Read the model definition and answer for the solid it produces. Units are mm, in the model's axes. Coordinates: 2 decimals unless noted, no trailing zeros. Write each loop counter-clockwise with the first axis right and the second up, starting at its lowest first coordinate (ties: lowest second). Pieces come first, ordered by that corner, then holes. Notation, with made-up numbers: (75.25, 21.5) -> (107.25, 21.5) arc R21 ccw to (107.25, 59.5) -> close; hole circle Ø8 at (31.5, 80). An arc over 180 degrees is marked (long way). Answer in a Markdown table with one row per item. Add a question column.
Item 1: Straight lines are drawn through the part: line 1 (Y direction, x = 54, z = 1.4); line 2 (Y direction, x = 134, z = 1.4); line 3 (Y direction, x = 182, z = 1.25). For each, find the intervals that lie inside material, in ascending order. Write a range as from..to.
Item 2: Section B-B on y = 72 is taken. Count the separate pieces of the cut face and the enclosed holes in it, then the cut area to 3 significant figures.
Item 3: Given pin 1 Ø1.5 at (x, z) = (89, 1) entering from -Y; pin 2 Ø1.5 at (y, z) = (1, 1.5) entering from +X; pin 3 Ø0.9 at (y, z) = (15.5, 1) entering from -X, each flat-ended and moving along its own axis, determine where each tip first touches the part or whether it passes through.
Item 4: For a pull along Y with two mould halves and no side action, classify faces 1 (the face through (108, 152, 3)), 2 (the face through (21.479, 35.966, 1.521)) as +Y half, -Y half, draft (parallel to the pull), parting line (faces both ways), or undercut.
Item 5: Section A-A on x = 77 is taken. Write down the section's boundary in (y, z).
Item 6: Section D-D on x = 165 is taken. Write down the section's boundary in (y, z), then the cut area to 3 significant figures.
```python
from build123d import *

# Parameters (mm, degrees)
SKETCH_W      = 220
SKETCH_H      = 300
PAD_DEPTH     = 3
SKETCH001_R   = 7.5
SKETCH001_R_2 = 4
SKETCH001_W   = 20
SKETCH001_H   = 3
SKETCH001_W_2 = 3
SKETCH001_H_2 = 20
SKETCH001_H_3 = 17
POCKET_DEPTH  = 5


with BuildPart() as part:
    # Sketch → Pad (new body)
    with BuildSketch(Plane.XY):
        with Locations((110, 150)):
            Rectangle(SKETCH_W, SKETCH_H)
    extrude(amount=PAD_DEPTH)

    # Sketch001 (on Face6 of Pad) → Pocket (cut)
    with BuildSketch(Plane.XY.offset(3)):
        with Locations((33, 72)):
            Circle(SKETCH001_R)
        with Locations((55, 72)):
            Circle(SKETCH001_R)
        with Locations((77, 72)):
            Circle(SKETCH001_R)
        with Locations((99, 72)):
            Circle(SKETCH001_R)
        with Locations((121, 72)):
            Circle(SKETCH001_R)
        with Locations((143, 72)):
            Circle(SKETCH001_R)
        with Locations((165, 72)):
            Circle(SKETCH001_R)
        with Locations((187, 72)):
            Circle(SKETCH001_R)
        with Locations((22, 48)):
            Circle(SKETCH001_R_2)
        with Locations((38, 48)):
            Circle(SKETCH001_R_2)
        with Locations((54, 48)):
            Circle(SKETCH001_R_2)
        with Locations((70, 48)):
            Circle(SKETCH001_R_2)
        with Locations((86, 48)):
            Circle(SKETCH001_R_2)
        with Locations((102, 48)):
            Circle(SKETCH001_R_2)
        with Locations((118, 48)):
            Circle(SKETCH001_R_2)
        with Locations((134, 48)):
            Circle(SKETCH001_R_2)
        with Locations((150, 48)):
            Circle(SKETCH001_R_2)
        with Locations((166, 48)):
            Circle(SKETCH001_R_2)
        with Locations((182, 48)):
            Circle(SKETCH001_R_2)
        with Locations((198, 48)):
            Circle(SKETCH001_R_2)
        with Locations((22, 32)):
            Circle(SKETCH001_R_2)
        with Locations((38, 32)):
            Circle(SKETCH001_R_2)
        with Locations((54, 32)):
            Circle(SKETCH001_R_2)
        with Locations((70, 32)):
            Circle(SKETCH001_R_2)
        with Locations((86, 32)):
            Circle(SKETCH001_R_2)
        with Locations((102, 32)):
            Circle(SKETCH001_R_2)
        with Locations((118, 32)):
            Circle(SKETCH001_R_2)
        with Locations((134, 32)):
            Circle(SKETCH001_R_2)
        with Locations((150, 32)):
            Circle(SKETCH001_R_2)
        with Locations((166, 32)):
            Circle(SKETCH001_R_2)
        with Locations((182, 32)):
            Circle(SKETCH001_R_2)
        with Locations((198, 32)):
            Circle(SKETCH001_R_2)
        with Locations((22, 16)):
            Circle(SKETCH001_R_2)
        with Locations((38, 16)):
            Circle(SKETCH001_R_2)
        with Locations((54, 16)):
            Circle(SKETCH001_R_2)
        with Locations((70, 16)):
            Circle(SKETCH001_R_2)
        with Locations((86, 16)):
            Circle(SKETCH001_R_2)
        with Locations((102, 16)):
            Circle(SKETCH001_R_2)
        with Locations((118, 16)):
            Circle(SKETCH001_R_2)
        with Locations((134, 16)):
            Circle(SKETCH001_R_2)
        with Locations((150, 16)):
            Circle(SKETCH001_R_2)
        with Locations((166, 16)):
            Circle(SKETCH001_R_2)
        with Locations((182, 16)):
            Circle(SKETCH001_R_2)
        with Locations((198, 16)):
            Circle(SKETCH001_R_2)
        with Locations((10, 1.5)):
            Rectangle(SKETCH001_W, SKETCH001_H)
        with Locations((50, 1.5)):
            Rectangle(SKETCH001_W, SKETCH001_H)
        with Locations((90, 1.5)):
            Rectangle(SKETCH001_W, SKETCH001_H)
        with Locations((130, 1.5)):
            Rectangle(SKETCH001_W, SKETCH001_H)
        with Locations((170, 1.5)):
            Rectangle(SKETCH001_W, SKETCH001_H)
        with Locations((210, 1.5)):
            Rectangle(SKETCH001_W, SKETCH001_H)
        with Locations((10, 298.5)):
            Rectangle(SKETCH001_W, SKETCH001_H)
        with Locations((50, 298.5)):
            Rectangle(SKETCH001_W, SKETCH001_H)
        with Locations((90, 298.5)):
            Rectangle(SKETCH001_W, SKETCH001_H)
        with Locations((130, 298.5)):
            Rectangle(SKETCH001_W, SKETCH001_H)
        with Locations((170, 298.5)):
            Rectangle(SKETCH001_W, SKETCH001_H)
        with Locations((210, 298.5)):
            Rectangle(SKETCH001_W, SKETCH001_H)
        with Locations((1.5, 50)):
            Rectangle(SKETCH001_W_2, SKETCH001_H_2)
        with Locations((1.5, 90)):
            Rectangle(SKETCH001_W_2, SKETCH001_H_2)
        with Locations((1.5, 130)):
            Rectangle(SKETCH001_W_2, SKETCH001_H_2)
        with Locations((1.5, 170)):
            Rectangle(SKETCH001_W_2, SKETCH001_H_2)
        with Locations((1.5, 210)):
            Rectangle(SKETCH001_W_2, SKETCH001_H_2)
        with Locations((1.5, 250)):
            Rectangle(SKETCH001_W_2, SKETCH001_H_2)
        with Locations((218.5, 50)):
            Rectangle(SKETCH001_W_2, SKETCH001_H_2)
        with Locations((218.5, 90)):
            Rectangle(SKETCH001_W_2, SKETCH001_H_2)
        with Locations((218.5, 130)):
            Rectangle(SKETCH001_W_2, SKETCH001_H_2)
        with Locations((218.5, 170)):
            Rectangle(SKETCH001_W_2, SKETCH001_H_2)
        with Locations((218.5, 210)):
            Rectangle(SKETCH001_W_2, SKETCH001_H_2)
        with Locations((218.5, 250)):
            Rectangle(SKETCH001_W_2, SKETCH001_H_2)
        with Locations((1.5, 11.51)):
            Rectangle(SKETCH001_W_2, SKETCH001_H_3)
        with Locations((1.5, 288.5)):
            Rectangle(SKETCH001_W_2, SKETCH001_H_3)
        with Locations((218.5, 288.5)):
            Rectangle(SKETCH001_W_2, SKETCH001_H_3)
        with Locations((218.5, 11.51)):
            Rectangle(SKETCH001_W_2, SKETCH001_H_3)
    extrude(amount=-POCKET_DEPTH, mode=Mode.SUBTRACT)


solid = part.part
```
Results below:
| question | item | result |
|---|---|---|
| 1 | line 1 | y = 3..12, 20..28, 36..44, 52..64.57, 79.43..297 |
| 1 | line 2 | y = 3..12, 20..28, 36..44, 52..297 |
| 1 | line 3 | y = 0..12, 20..28, 36..44, 52..66.41, 77.59..300 |
| 2 | separate pieces | 9 |
| 2 | enclosed holes | 0 |
| 2 | area | 300 mm2 |
| 3 | pin 1 | stops at y = 3 |
| 3 | pin 2 | stops at x = 200 |
| 3 | pin 3 | stops at x = 3 |
| 4 | face 1 | draft |
| 4 | face 2 | undercut |
| 5 | outline | (0, 0) -> (64.5, 0) -> (64.5, 3) -> (0, 3) -> close; (79.5, 0) -> (300, 0) -> (300, 3) -> (79.5, 3) -> close |
| 6 | outline | (3, 0) -> (12.13, 0) -> (12.13, 3) -> (3, 3) -> close; (19.87, 0) -> (28.13, 0) -> (28.13, 3) -> (19.87, 3) -> close; (35.87, 0) -> (44.13, 0) -> (44.13, 3) -> (35.87, 3) -> close; (51.87, 0) -> (64.5, 0) -> (64.5, 3) -> (51.87, 3) -> close; (79.5, 0) -> (297, 0) -> (297, 3) -> (79.5, 3) -> close |
| 6 | area | 767 mm2 |
